from build123d import *

# Parameters (mm, degrees)
SKETCH1_W           = 60
SKETCH1_H           = 25
BOSS_EXTRUDE1_DEPTH = 82
CUT_EXTRUDE7_DEPTH  = 3.5
SKETCH50_W          = 52.5
SKETCH50_H          = 4.5
CUT_EXTRUDE9_DEPTH  = 80.605527446
SKETCH51_W          = 9.5
SKETCH51_H          = 34
BOSS_EXTRUDE2_DEPTH = 3
SKETCH52_W          = 43
SKETCH52_H          = 34
CUT_EXTRUDE10_DEPTH = 10
CUT_EXTRUDE11_DEPTH = 4
CUT_EXTRUDE12_DEPTH = 4
CUT_EXTRUDE13_DEPTH = 3.5
CUT_EXTRUDE14_DEPTH = 3.5
CUT_EXTRUDE15_DEPTH = 88.408752422
CUT_EXTRUDE16_DEPTH = 59.086142926
CUT_EXTRUDE17_DEPTH = 88.408752422
CUT_EXTRUDE18_DEPTH = 15
HOLE1_D             = 4.2
HOLE2_D             = 4.4
HOLE3_D             = 4.4
HOLE4_D             = 8
SKETCH125_W         = 5.08
SKETCH125_H         = 27.94
CUT_EXTRUDE19_DEPTH = 3.556
SKETCH126_W         = 9.92
SKETCH126_H         = 28.017689761
CUT_EXTRUDE20_DEPTH = 20.066
CUT_EXTRUDE21_DEPTH = 80.605527446


with BuildPart() as part:
    # Sketch1 → Boss-Extrude1 (new body)
    with BuildSketch(Plane(origin=(-39, 0, 0), x_dir=(0, -1, 0), z_dir=(-1, 0, 0))):
        with Locations((0, 17.3)):
            Rectangle(SKETCH1_W, SKETCH1_H)
        with BuildLine():
            Line((22, 15.753862534), (18.978772839, 18.882434844))
            ThreePointArc((18.978772839, 18.882434844), (22, 26), (25.021227161, 18.882434844))
            Line((25.021227161, 18.882434844), (22, 15.753862534))
        make_face(mode=Mode.SUBTRACT)
        with BuildLine():
            Line((-18.978772839, 18.882434844), (-22, 15.753862534))
            Line((-22, 15.753862534), (-25.021227161, 18.882434844))
            ThreePointArc((-25.021227161, 18.882434844), (-22, 26), (-18.978772839, 18.882434844))
        make_face(mode=Mode.SUBTRACT)
    extrude(amount=-BOSS_EXTRUDE1_DEPTH)

    # Sketch39 → Cut-Extrude7 (cut)
    with BuildSketch(Plane(origin=(0, 0, 4.8), x_dir=(-1, 0, 0), z_dir=(0, 0, -1))):
        Polygon((-28, 14), (-28, -14), (-25, -14), (-25, -30), (39, -30), (39, 30), (-25, 30), (-25, 14), align=None)
    extrude(amount=-CUT_EXTRUDE7_DEPTH, mode=Mode.SUBTRACT)

    # Sketch50 → Cut-Extrude9 (cut, through all)
    with BuildSketch(Plane.XZ.offset(30)):
        with Locations((-12.75, 10.55)):
            Rectangle(SKETCH50_W, SKETCH50_H)
    extrude(amount=-CUT_EXTRUDE9_DEPTH, mode=Mode.SUBTRACT)

    # Sketch51 → Boss-Extrude2 (add)
    with BuildSketch(Plane(origin=(0, 0, 12.8), x_dir=(-1, 0, 0), z_dir=(0, 0, -1))):
        with Locations((34.25, 0)):
            Rectangle(SKETCH51_W, SKETCH51_H)
    extrude(amount=BOSS_EXTRUDE2_DEPTH)

    # Sketch52 → Cut-Extrude10 (cut)
    with BuildSketch(Plane(origin=(0, 0, 12.8), x_dir=(-1, 0, 0), z_dir=(0, 0, -1))):
        with Locations((8, 0)):
            Rectangle(SKETCH52_W, SKETCH52_H)
    extrude(amount=-CUT_EXTRUDE10_DEPTH, mode=Mode.SUBTRACT)

    # Sketch63 → Cut-Extrude11 (cut)
    with BuildSketch(Plane(origin=(-29.5, 0, 0), x_dir=(0, 0, -1), z_dir=(1, 0, 0))):
        Polygon((-22.8, 4.892671517), (-19.15, 2.785343035), (-15.559049818, 4.858579089), (-13.34154355, 7), (-15.559049818, 9.141420911), (-19.15, 11.214656965), (-22.8, 9.107328483), align=None)
    extrude(amount=-CUT_EXTRUDE11_DEPTH, mode=Mode.SUBTRACT)

    # Sketch75 → Cut-Extrude12 (cut)
    with BuildSketch(Plane(origin=(-29.5, 0, 0), x_dir=(0, 0, -1), z_dir=(1, 0, 0))):
        Polygon((-15.559049818, -4.858579089), (-19.15, -2.785343035), (-22.8, -4.892671517), (-22.8, -9.107328483), (-19.15, -11.214656965), (-15.559049818, -9.141420911), (-13.34154355, -7), align=None)
    extrude(amount=-CUT_EXTRUDE12_DEPTH, mode=Mode.SUBTRACT)

    # Sketch76 → Cut-Extrude13 (cut)
    with BuildSketch(Plane(origin=(0, 0, 4.8), x_dir=(-1, 0, 0), z_dir=(0, 0, -1))):
        with BuildLine():
            Line((-25, -18.693747285), (-25, -14))
            Line((-25, -14), (-29.099342077, -14))
            ThreePointArc((-29.099342077, -14), (-27.525501185, -16.762445769), (-25, -18.693747285))
        make_face()
    extrude(amount=-CUT_EXTRUDE13_DEPTH, mode=Mode.SUBTRACT)

    # Sketch77 → Cut-Extrude14 (cut)
    with BuildSketch(Plane(origin=(0, 0, 4.8), x_dir=(-1, 0, 0), z_dir=(0, 0, -1))):
        with BuildLine():
            Line((-29.099342077, 14), (-25, 14))
            Line((-25, 14), (-25, 18.693747285))
            ThreePointArc((-25, 18.693747285), (-27.525501185, 16.762445769), (-29.099342077, 14))
        make_face()
    extrude(amount=-CUT_EXTRUDE14_DEPTH, mode=Mode.SUBTRACT)

    # Sketch89 → Cut-Extrude15 (cut, through all)
    with BuildSketch(Plane(origin=(-33.5, 0, 0), x_dir=(0, 0, -1), z_dir=(1, 0, 0))):
        with BuildLine():
            Line((-15.982975613, 7), (-17.621751585, 8.582547561))
            ThreePointArc((-17.621751585, 8.582547561), (-21.35, 7), (-17.621751585, 5.417452439))
            Line((-17.621751585, 5.417452439), (-15.982975613, 7))
        make_face()
    extrude(amount=-CUT_EXTRUDE15_DEPTH, mode=Mode.SUBTRACT)

    # Sketch90 → Cut-Extrude16 (cut, through all)
    with BuildSketch(Plane.XY.offset(29.8)):
        with BuildLine():
            Line((-23.4, -2.2), (-20.981803131, -2.2))
            ThreePointArc((-20.981803131, -2.2), (-15.6, -9.699484522), (-6.414354323, -10.61052049))
            Line((-6.414354323, -10.61052049), (-5.205255888, -12.704740411))
            ThreePointArc((-5.205255888, -12.704740411), (-2.2, -13.509996299), (-1.394744112, -10.504740411))
            Line((-1.394744112, -10.504740411), (-2.603842546, -8.41052049))
            ThreePointArc((-2.603842546, -8.41052049), (1.2, 0), (-2.603842546, 8.41052049))
            Line((-2.603842546, 8.41052049), (-1.394744112, 10.504740411))
            ThreePointArc((-1.394744112, 10.504740411), (-2.2, 13.509996299), (-5.205255888, 12.704740411))
            Line((-5.205255888, 12.704740411), (-6.414354323, 10.61052049))
            ThreePointArc((-6.414354323, 10.61052049), (-15.6, 9.699484522), (-20.981803131, 2.2))
            Line((-20.981803131, 2.2), (-23.4, 2.2))
            ThreePointArc((-23.4, 2.2), (-25.6, 0), (-23.4, -2.2))
        make_face()
    extrude(amount=-CUT_EXTRUDE16_DEPTH, mode=Mode.SUBTRACT)

    # Sketch103 → Cut-Extrude17 (cut, through all)
    with BuildSketch(Plane(origin=(-33.5, 0, 0), x_dir=(0, 0, -1), z_dir=(1, 0, 0))):
        with BuildLine():
            Line((-17.621751585, -8.582547561), (-15.982975613, -7))
            Line((-15.982975613, -7), (-17.621751585, -5.417452439))
            ThreePointArc((-17.621751585, -5.417452439), (-21.35, -7), (-17.621751585, -8.582547561))
        make_face()
    extrude(amount=-CUT_EXTRUDE17_DEPTH, mode=Mode.SUBTRACT)

    # Sketch116 → Cut-Extrude18 (cut)
    with BuildSketch(Plane(origin=(0, 0, 8.3), x_dir=(-1, 0, 0), z_dir=(0, 0, -1))):
        Polygon((-19.5, 4.214656965), (-23.090950182, 2.141420911), (-23.090950182, -2.141420911), (-19.5, -4.214656965), (-15.85, -2.107328483), (-15.85, 2.107328483), align=None)
    extrude(amount=-CUT_EXTRUDE18_DEPTH, mode=Mode.SUBTRACT)

    # Hole1 (through all)
    with Locations(Plane(origin=(0, 0, 23.3), x_dir=(-1, 0, 0), z_dir=(0, 0, -1))):
        with Locations((-19.470475091, 0.017046214)):
            Hole(HOLE1_D / 2)

    # Hole2 (through all)
    with Locations(Plane(origin=(0, 0, 8.3), x_dir=(-1, 0, 0), z_dir=(0, 0, -1))):
        with Locations((-21.5, 11.5)):
            Hole(HOLE2_D / 2)

    # Hole3 (through all)
    with Locations(Plane(origin=(0, 0, 8.3), x_dir=(-1, 0, 0), z_dir=(0, 0, -1))):
        with Locations((-21.5, -11.5)):
            Hole(HOLE3_D / 2)

    # Hole4 (through all)
    with Locations(Plane(origin=(0, 0, 9.8), x_dir=(-1, 0, 0), z_dir=(0, 0, -1))):
        with Locations((39, 0)):
            Hole(HOLE4_D / 2)

    # Sketch125 → Cut-Extrude19 (cut)
    with BuildSketch(Plane(origin=(0, 0, 4.8), x_dir=(-1, 0, 0), z_dir=(0, 0, -1))):
        with Locations((-40.46, 0)):
            Rectangle(SKETCH125_W, SKETCH125_H)
    extrude(amount=-CUT_EXTRUDE19_DEPTH, mode=Mode.SUBTRACT)

    # Sketch126 → Cut-Extrude20 (cut)
    with BuildSketch(Plane(origin=(0, 0, 4.8), x_dir=(-1, 0, 0), z_dir=(0, 0, -1))):
        with Locations((-32.96, 0.008844881)):
            Rectangle(SKETCH126_W, SKETCH126_H)
    extrude(amount=-CUT_EXTRUDE20_DEPTH, mode=Mode.SUBTRACT)

    # Sketch128 → Cut-Extrude21 (cut, through all)
    with BuildSketch(Plane(origin=(0, 30, 0), x_dir=(1, 0, 0), z_dir=(0, 1, 0))):
        with BuildLine():
            Line((30.094465156, -10.583890742), (33.094, -7.477781484))
            Line((33.094, -7.477781484), (36.093534844, -10.583890742))
            ThreePointArc((36.093534844, -10.583890742), (33.094, -18.008), (30.094465156, -10.583890742))
        make_face()
    extrude(amount=-CUT_EXTRUDE21_DEPTH, mode=Mode.SUBTRACT)


solid = part.part
CAD build for the part. Positions are in the model's coordinates, mm. A direction names the side the tool comes from. Round coordinates to 2 decimals unless told otherwise and drop trailing zeros. Order: outer loops, then holes, each group sorted by start corner. A loop starts at its lowest first (then second) coordinate and runs counter-clockwise, first axis right, second up. Notation, with made-up numbers: (53, 52.25) -> (107, 52.25) arc R20 ccw to (107, 91.25) -> close; hole circle Ø7 at (-12.5, 21.5). An arc over 180 degrees is marked (long way). Write item = value, one per line. Start each with the question number.
(1) Cut at C-C, the plane y = 23. List the corners of the cut face in (x, z), then the cut area to 3 significant figures.
(2) Probe line 1 (X direction, y = 2, z = 9.75); line 2 (X direction, y = 20.75, z = 13.69); line 3 (Y direction, x = 25.5, z = 19.5). List the from-to ranges inside material, lowest first. Write a range as [from, to].
(3) Which spindle directions (+Z, -Z, +X, -X, +Y, -Y) get a long thin tool onto all of the face, cutting with end or side? Do faces 1 (the flat face through (-13, -24, 12.8)), 2 (the flat face through (-31.472, -3.824, 20.949)), 3 (the flat face through (31.573, 22.121, 9.053)). Say none if no direction does.
(4) Pull direction Z, two halves, no side cores. Call faces 4 (the flat face through (-5.801, 11.672, 26.349)), 5 (the flat face through (-13, 23, 12.8)), 6 (the flat face through (-31.472, 10.164, 17.329)): released by +Z, released by -Z, zero draft, split by the parting line, or undercut.
(5) Cut at B-B, the plane z = 27.75. List the corners of the cut face in (x, y).
(6) Cut at A-A, the plane x = -13. List the corners of the cut face in (y, z).
(7) Cut at D-D, the plane y = -15. List the corners of the cut face in (x, z), then the cut area to 3 significant figures.
(8) Pin check, flat tips, straight feed: P1, Ø1, axis at x = 6.5, y = 7, coming from the -Z side; P2, Ø4.5, axis at y = 0, z = 17.5, coming from the -X side; P3, Ø5.5, axis at x = 21.5, y = -11.5, coming from the +Z side; P4, Ø4, axis at y = 22.5, z = 6, coming from the -X side. Stop position of each tip, or through.
Model answer:
q1.outline = (-39, 12.8) -> (13.5, 12.8) -> (13.5, 8.3) -> (25, 8.3) -> (25, 4.8) -> (43, 4.8) -> (43, 16.79) -> (36.1, 16.79) arc R4.32 cw to (36.09, 10.58) -> (33.09, 7.48) -> (30.09, 10.58) arc R4.32 cw to (30.09, 16.79) -> (-39, 16.79) -> close; (-39, 25.88) -> (43, 25.88) -> (43, 29.8) -> (-39, 29.8) -> close
q1.area = 787 mm2
q2.line_1 = [13.5, 15.85], [23.09, 28], [37.92, 43]
q2.line_2 = [-39, 28.78], [37.41, 43]
q2.line_3 = [-30, -25.51], [-18.49, 18.49], [25.51, 30]
q3.face_1 = -Z, -X, -Y
q3.face_2 = none
q3.face_3 = +Y, -Y
q4.face_4 = zero draft
q4.face_5 = released by -Z
q4.face_6 = undercut
q5.outline = (-39, -30) -> (43, -30) -> (43, 30) -> (-39, 30) -> (-39, 4) arc R4 cw to (-39, -4) -> close; hole (-23.4, -2.2) -> (-20.98, -2.2) arc R11.2 ccw to (-6.41, -10.61) -> (-5.21, -12.7) arc R2.2 ccw to (-1.39, -10.5) -> (-2.6, -8.41) arc R11.2 ccw to (-2.6, 8.41) -> (-1.39, 10.5) arc R2.2 ccw to (-5.21, 12.7) -> (-6.41, 10.61) arc R11.2 ccw to (-20.98, 2.2) -> (-23.4, 2.2) arc R2.2 ccw to start; hole circle Ø4.2 at (19.47, 0.02); hole circle Ø4.4 at (21.5, -11.5); hole circle Ø4.4 at (21.5, 11.5)
q6.outline = (-30, 12.8) -> (-17, 12.8) -> (-17, 22.8) -> (-10.79, 22.8) -> (-10.79, 29.8) -> (-30, 29.8) -> close; (10.79, 22.8) -> (17, 22.8) -> (17, 12.8) -> (30, 12.8) -> (30, 29.8) -> (10.79, 29.8) -> close; hole (-25.02, 18.88) -> (-22, 15.75) -> (-18.98, 18.88) arc R4.2 ccw (long way) to start; hole (18.98, 18.88) -> (22, 15.75) -> (25.02, 18.88) arc R4.2 ccw (long way) to start
q7.outline = (-39, 9.8) -> (-29.5, 9.8) -> (-29.5, 22.8) -> (13.5, 22.8) -> (13.5, 8.3) -> (28.69, 8.3) -> (28.69, 4.8) -> (43, 4.8) -> (43, 29.8) -> (-39, 29.8) -> close; hole (30.09, 10.58) -> (33.09, 7.48) -> (36.09, 10.58) arc R4.32 ccw (long way) to start
q7.area = 1,110 mm2
q8.P1 = 22.8
q8.P2 = -35.69
q8.P3 = 29.8
q8.P4 = 25
